Autodesk Inventor part; units mm, degrees
ref_plane "YZ Plane" through (0, 0, 0) normal (1, 0, 0) x (0, 1, 0)
ref_plane "XZ Plane" through (0, 0, 0) normal (0, 1, 0) x (-1, 0, 0)
ref_plane "XY Plane" through (0, 0, 0) normal (0, 0, 1) x (1, 0, 0)
sketch "Sketch1" plane through (0, 0, 0) normal (0, 1, 0) x (-1, 0, 0)
  line L0 (0, 0) -> (-12922.0343, 0) construction
  line L1 (0, 0) -> (-12360.1465, -3311.8913) construction
  line L2 (0, 0) -> (13412.8311, 0) construction
  line L3 (-4192.3928, 50) -> (-5417.1104, 50)
  line L4 (-4036.5995, -1133.3674) -> (-5219.5859, -1450.3476)
  line L5 (-5417.1104, 12) -> (-5229.4211, -1413.6425)
  line L6 (-4041.5281, -1095.9314) -> (-4187.39, 12)
  line L7 (0, 0) -> (-4114.4962, -541.6837) construction
  line L8 (0, 0) -> (4150, 0) construction
  line L9 (-5378.7825, 12) -> (-4225.7179, 12)
  line L10 (-4225.7179, 12) -> (-4078.6242, -1105.2874)
  line L11 (-4078.6242, -1105.2874) -> (-5192.3991, -1403.7225)
  line L12 (-5192.3991, -1403.7225) -> (-5378.7825, 12)
  line L13 (-5378.7825, 12) -> (-5445.5914, 12) construction
  line L14 (-5417.1104, 12) -> (-5417.1104, 50)
  line L15 (-4225.7179, 12) -> (-4187.39, 12) construction
  line L16 (-4187.39, 12) -> (-4187.39, 50)
  line L17 (-4187.39, 50) -> (-4192.3928, 50)
  line L18 (-4076.4449, -1105.2874) -> (-4041.5281, -1095.9314) construction
  line L19 (-4041.5281, -1095.9314) -> (-4031.8389, -1132.0918)
  line L20 (-4031.8389, -1132.0918) -> (-4036.5995, -1133.3674)
  line L21 (-5192.3991, -1403.7225) -> (-5229.4211, -1413.6425) construction
  line L22 (-5229.4211, -1413.6425) -> (-5219.5859, -1450.3476)
  dimension "d0" = 165
  dimension "d3" = 50
  dimension "d4" = 50
  dimension "d6" = 4150
  dimension "d7" = 172.5
  dimension "d10" = 38
extrude "Extrusion2" add sketch "Sketch1" along normal blind 114
sketch "Sketch2" plane through (0, 114, 0) normal (0, 1, 0) x (1, 0, 0)
  line L0 (4225.7179, -12) -> (4078.6242, 1105.2874)
  line L1 (4041.5281, 1095.9314) -> (4187.39, -12)
  line L2 (4187.39, -12) -> (4187.39, -50)
  line L3 (4078.6242, 1105.2874) -> (4041.5281, 1095.9314)
  line L4 (4225.7179, -12) -> (4187.39, -12)
  point P0 (0, 0)
extrude "Extrusion3" cut sketch "Sketch2" against normal blind 1
sketch "Sketch3" plane through (0, 114, 0) normal (0, 1, 0) x (1, 0, 0)
  line L0 (5192.3991, 1403.7225) -> (5378.7825, -12)
  line L1 (5417.1104, -50) -> (5417.1104, -12)
  line L2 (5417.1104, -12) -> (5229.4211, 1413.6425)
  line L3 (4031.8389, 1132.0918) -> (4041.5281, 1095.9314)
  line L4 (5192.3991, 1403.7225) -> (5229.4211, 1413.6425)
  line L5 (5378.7825, -12) -> (5417.1104, -12)
  point P0 (0, 0)
extrude "Extrusion4" cut sketch "Sketch3" against normal blind 1
properties part number "panelCflat" material "Wood (Birch)"
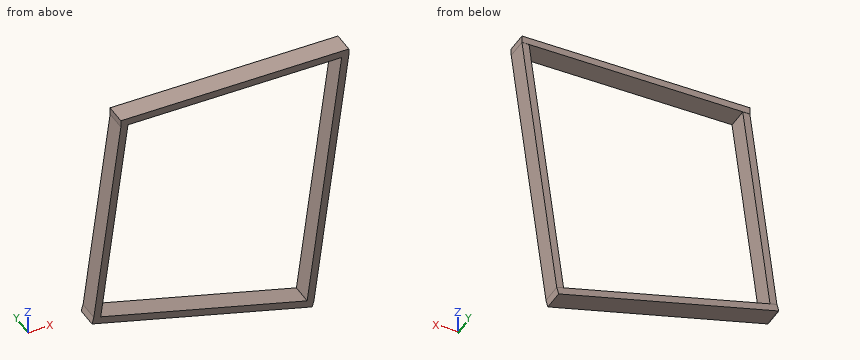
Geometry: final body of the model. Coordinates: model frame, mm. Round coordinates to 2 decimals unless told otherwise and drop trailing zeros. Loops run counter-clockwise (first coordinate to the right, second up) from the corner with the lowest first, then second, coordinate; pieces in that order, holes last.
Q1. Section A-A on y = 50. Return loops of the section in (x, z).
Q2. Section C-C on x = 4775.5. Return loops of the section in (y, z), plus the area to 3 significant figures.
Q3. Pin query (flat end, axial travel): P1, Ø1, axis at y = 40.5, z = -664, coming from the +X side; P2, Ø8, axis at y = 71.5, z = -1053, coming from the +X side; P3, Ø3, axis at x = 4329.5, y = 59, coming from the -Z side. Return the tip coordinate at first contact, or that it passes through.
Q4. Section B-B on z = -192.5. Return loops of the section in (x, y), plus the area to 3 significant figures.
Q5. Material intervals for L1, parallel to X at y = 70.5, z = -482; L2, parallel to Z at x = 4468, y = 97; L3, parallel to X at y = 47.5, z = -986, sorted ascending.
Evaluation:
1. outline: (4031.84, -1132.09) - (4036.6, -1133.37) - (5219.59, -1450.35) - (5229.42, -1413.64) - (5417.11, 12) - (5417.11, 50) - (4187.39, 50) - (4187.39, 12) - (4041.53, -1095.93) - close; hole (4078.62, -1105.29) - (5192.4, -1403.72) - (5378.78, 12) - (4225.72, 12) - close
2. outline: (0, -1331.36) - (114, -1331.36) - (114, -1292.01) - (0, -1292.01) - close; (0, 12) - (114, 12) - (114, 50) - (0, 50) - close
2. area: 8,820 mm2
3. P1: stops at x = 5328.18
3. P2: stops at x = 5277.43
3. P3: stops at z = -1212.25
4. outline: (4160.47, 0) - (4198.79, 0) - (4198.79, 113) - (4160.47, 113) - close; (5351.86, 0) - (5390.19, 0) - (5390.19, 113) - (5351.86, 113) - close
4. area: 8,660 mm2
5. L1: x = 4122.35 to 4160.68, 5313.75 to 5352.07
5. L2: z = -1248.96 to -1209.62, 12 to 50
5. L3: x = 4056 to 4094.33, 5247.39 to 5285.72
